from build123d import *

# Parameters (mm, degrees)
CHAMFER1_SIZE      = 0.875
CUT_EXTRUDE1_START = -6.000000232
CUT_EXTRUDE1_DEPTH = 7.000000232
FILLET2_R          = 0.6


with BuildPart() as part:
    # Sketch1 → Revolve1 (revolve)
    with BuildSketch(Plane(origin=(0, 0, 0), x_dir=(0, 0, -1), z_dir=(1, 0, 0)), mode=Mode.PRIVATE) as revolve1_sk:
        Polygon((0, 9), (-12, 9), (-12, 0), (180, 0), (180, 6), (0, 6), align=None)
    revolve(revolve1_sk.sketch.rotate(Axis((0, 0, 12), (0, 0, -1)), 180), axis=Axis((0, 0, 12), (0, 0, -1)))

    # Sketch7 → Cut-Revolve2 (revolve, cut)
    with BuildSketch(Plane(origin=(0, 0, 0), x_dir=(0, 0, -1), z_dir=(1, 0, 0)), mode=Mode.PRIVATE) as cut_revolve2_sk:
        Polygon((-12, 0), (-12, 5), (-6, 5), (-3.113248654, 0), align=None)
    revolve(cut_revolve2_sk.sketch.rotate(Axis((0, 0, 12), (0, 0, -1)), 90), axis=Axis((0, 0, 12), (0, 0, -1)), mode=Mode.SUBTRACT)

    # Chamfer1
    chamfer1_edges = [part.edges().sort_by_distance(p)[0] for p in [
        (0, 9, 12),
        (0, 6, -180),
    ]]
    chamfer(chamfer1_edges, length=CHAMFER1_SIZE)

    # Cut-Extrude1: read off the stored shape, not the designer's step
    # Cut-Extrude1 outline → Cut-Extrude1 (cut)
    with BuildSketch(Plane.XY.offset(12).offset(CUT_EXTRUDE1_START)):
        with BuildLine():
            Line((5, 0), (5, 2.886751346))
            Line((5, 2.886751346), (2.500000011, 4.330127013))
            ThreePointArc((2.500000011, 4.330127013), (4.330127022, 2.499999995), (5, 0))
        make_face()
        with BuildLine():
            ThreePointArc((-2.500000011, 4.330127013), (0, 5), (2.500000011, 4.330127013))
            Line((2.500000011, 4.330127013), (0, 5.773502692))
            Line((0, 5.773502692), (-2.500000011, 4.330127013))
        make_face()
        with BuildLine():
            Line((5, -2.886751346), (5, 0))
            ThreePointArc((5, 0), (4.330127007, -2.500000021), (2.499999959, -4.330127043))
            Line((2.499999959, -4.330127043), (5, -2.886751346))
        make_face()
        with BuildLine():
            ThreePointArc((-5, 0), (-4.330127022, 2.499999995), (-2.500000011, 4.330127013))
            Line((-2.500000011, 4.330127013), (-5, 2.886751346))
            Line((-5, 2.886751346), (-5, 0))
        make_face()
        with BuildLine():
            Line((0, -5.773502692), (2.499999959, -4.330127043))
            ThreePointArc((2.499999959, -4.330127043), (-6e-08, -5), (-2.500000063, -4.330126983))
            Line((-2.500000063, -4.330126983), (0, -5.773502692))
        make_face()
        with BuildLine():
            ThreePointArc((-2.500000063, -4.330126983), (-4.330127037, -2.499999969), (-5, 0))
            Line((-5, 0), (-5, -2.886751346))
            Line((-5, -2.886751346), (-2.500000063, -4.330126983))
        make_face()
    extrude(amount=CUT_EXTRUDE1_DEPTH, mode=Mode.SUBTRACT)

    # Cut-Extrude1 2 outline → Cut-Extrude1 2 (revolve)
    with BuildSketch(Plane.XZ):
        Polygon((5.773502705, 6.446581995), (4.9999999, 5.999999942), (5.773502692, 5.999999768), align=None)
    revolve(axis=Axis((0, 0, 0), (0, 0, 1)))

    # Sketch9 → Cut-Revolve3 (revolve, cut)
    with BuildSketch(Plane(origin=(0, 0, 0), x_dir=(0, 0, -1), z_dir=(1, 0, 0))):
        Polygon((-12.5, 6.639528096), (-12.5, 5), (-11.553418013, 5), align=None)
    revolve(axis=Axis((0, 0, 12), (0, 0, -1)), mode=Mode.SUBTRACT)

    # Fillet2
    fillet2_edges = [part.edges().sort_by_distance(p)[0] for p in [
        (0, 6, 0),
    ]]
    fillet(fillet2_edges, radius=FILLET2_R)


solid = part.part
Check sheet for the modelled part. Datum: model origin and axes. Units: mm. A direction names the side the tool comes from. Give positions to 0.01 mm unless a question says otherwise; leave off trailing zeros. Write each loop counter-clockwise with the first axis right and the second up, starting at its lowest first coordinate (ties: lowest second). Pieces come first, ordered by that corner, then holes. Notation, with made-up numbers: (80.5, -9) -> (116.5, -9) arc R19 ccw to (116.5, 7) -> close; hole circle Ø5 at (38, -30). An arc over 180 degrees is marked (long way). Use one line per item in the form item = value. Start each with the question number.
1. Thickness scan on line 1 along Z through (x, y) = (-1.5, 7); line 2 along Z through (x, y) = (4.75, -1.75); line 3 along X through (y, z) = (0.25, -33). Record the ranges inside material, lowest first. Write a range as from..to.
2. Go/stop test with flat-tipped pins: P1, Ø8, axis at x = -1.5, z = -84, coming from the +Y side; P2, Ø1.5, axis at y = -7, z = -132, coming from the -X side; P3, Ø8, axis at y = 1.5, z = -57.5, coming from the +X side; P4, Ø10, axis at x = 0.5, z = -132, coming from the -Y side. Record where each tip stops, or that it passes through.
3. Mould release check, pull along Y, two halves, no side actions. Record for faces 1 (the flat face through (5, 0, 9)), 2 (the flat face through (-6, -2, 12)), 3 (the cylindrical face through (-6.083, 6.633, 5.64)): pulls with the +Y half, pulls with the -Y half, needs draft (parallel to the pull), parting line crosses it, or undercut.
4. Access from +Z, -Z, +X, -X, +Y, -Y to the whole of each face (thin tool, end or side, straight path). Record for faces 4 (the flat face through (-5, 0, 9)), 5 (the flat face through (0, 0, -180)), 6 (the cylindrical face through (-1.802, -5.723, -88.613)).
5. Section check A-A (z = -99.5). Record the cut outline in (x, y).
Conclusion:
q1.line_1 = 0..12
q1.line_2 = -180..6.04
q1.line_3 = -5.99..5.99
q2.P1 = 6
q2.P2 = through
q2.P3 = 6
q2.P4 = -6
q3.face_1 = undercut
q3.face_2 = needs draft
q3.face_3 = parting line crosses it
q4.face_4 = +Z
q4.face_5 = -Z, +X, -X, +Y, -Y
q4.face_6 = -Z
q5.outline = circle Ø12 at (0, 0)
